Here's how the part is built. I have some questions about the finished solid (model axes, mm). Face numbers are marked on the shaded views. A direction names the side the tool comes from. Coordinates: 2 decimals unless noted, no trailing zeros. Loops run counter-clockwise (first coordinate to the right, second up) from the corner with the lowest first, then second, coordinate; pieces in that order, holes last. Notation, with made-up numbers: (87, -23) -> (109, -23) arc R19 ccw to (109, -8) -> close; hole circle Ø11 at (-16, 45.5). An arc over 180 degrees is marked (long way). Answer as a JSON object with one key per item and string values. Group by question number.
Q1. I want a section at D-D on y = -2.25. Write out the boundary of the cut face in (x, z).
Q2. I need wall thicknesses on line 1 (X direction, y = 0.5, z = 2.5); line 2 (X direction, y = -2.75, z = 1.45); line 3 (Y direction, x = 4.9, z = 1.7) (3 decimals). Which ranges of each line are inside material? Lowest first, please.
Q3. Thinking about a two-plate mould opening in X: for the marked faces 1, 2 and 3, which applies, released by +X, released by -X, zero draft, split by the parting line, or undercut?
Q4. I want a section at C-C on z = 1.2. Write out the boundary of the cut face in (x, y) (3 decimals), then the cut area to 3 significant figures.
Q5. I want a section at A-A on y = 0.95. Write out the boundary of the cut face in (x, z) (3 decimals).
Q6. I want a section at B-B on x = -4.9. Write out the boundary of the cut face in (y, z) (3 decimals), then the cut area to 4 significant figures.
Q7. I'm going to push flat-ended pins straight in: pin 1 (3 mm diameter, centred on x = 4.9, y = 0.95, fed in from +Z); pin 2 (1.6 mm diameter, centred on x = 0, z = 1, fed in from -Y). Where does each tip first touch, or does it pass through?
Q8. On a 3-axis mill with a long thin cutter (end or side, diameter ignored), from which of +Z, -Z, +X, -X, +Y, -Y can I reach the whole of each face in a straight line? I mean the marked faces 4 and 5. Say none if no direction works.
```python
from build123d import *

# Parameters (mm, degrees)
SKETCH1_W           = 20.2
SKETCH1_H           = 7.4
SKETCH1_R           = 1.725
BOSS_EXTRUDE1_DEPTH = 3
SKETCH2_W           = 2
SKETCH2_H           = 6
CUT_EXTRUDE1_DEPTH  = 3
FILLET1_R           = 1


with BuildPart() as part:
    # Sketch1 → Boss-Extrude1 (new body)
    with BuildSketch(Plane.XY):
        Rectangle(SKETCH1_W, SKETCH1_H)
        with Locations((-4.9, 0.95)):
            Circle(SKETCH1_R, mode=Mode.SUBTRACT)
        with Locations((4.9, 0.95)):
            Circle(SKETCH1_R, mode=Mode.SUBTRACT)
    extrude(amount=BOSS_EXTRUDE1_DEPTH)

    # Sketch2 → Cut-Extrude1 (cut)
    with BuildSketch(Plane.XY.offset(3)):
        with Locations((0, -0.7)):
            Rectangle(SKETCH2_W, SKETCH2_H)
    extrude(amount=-CUT_EXTRUDE1_DEPTH, mode=Mode.SUBTRACT)

    # Fillet1
    fillet1_edges = [part.edges().sort_by_distance(p)[0] for p in [
        (-10.1, 3.7, 1.5),
        (10.1, 3.7, 1.5),
    ]]
    fillet(fillet1_edges, radius=FILLET1_R)


solid = part.part
```
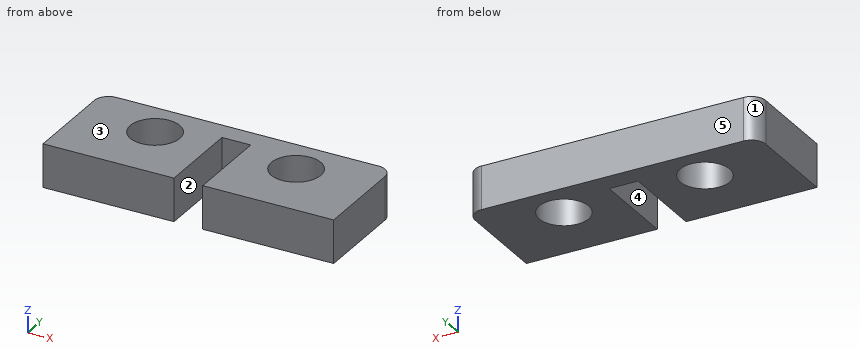
Result set:
{
 "1": {"outline": "(-10.1, 0) -> (-1, 0) -> (-1, 3) -> (-10.1, 3) -> close; (1, 0) -> (10.1, 0) -> (10.1, 3) -> (1, 3) -> close"},
 "2": {"line 1": "x = -10.1 to -6.57, -3.23 to -1, 1 to 3.23, 6.57 to 10.1", "line 2": "x = -10.1 to -1, 1 to 10.1", "line 3": "y = -3.7 to -0.775, 2.675 to 3.7"},
 "3": {"face 1": "released by -X", "face 2": "undercut", "face 3": "zero draft"},
 "4": {"outline": "(-10.1, -3.7) -> (-1, -3.7) -> (-1, 2.3) -> (1, 2.3) -> (1, -3.7) -> (10.1, -3.7) -> (10.1, 2.7) arc R1 ccw to (9.1, 3.7) -> (-9.1, 3.7) arc R1 ccw to (-10.1, 2.7) -> close; hole circle Ø3.45 at (-4.9, 0.95); hole circle Ø3.45 at (4.9, 0.95)", "area": "118 mm²"},
 "5": {"outline": "(-10.1, 0) -> (-6.625, 0) -> (-6.625, 3) -> (-10.1, 3) -> close; (-3.175, 0) -> (-1, 0) -> (-1, 3) -> (-3.175, 3) -> close; (1, 0) -> (3.175, 0) -> (3.175, 3) -> (1, 3) -> close; (6.625, 0) -> (10.1, 0) -> (10.1, 3) -> (6.625, 3) -> close"},
 "6": {"outline": "(-3.7, 0) -> (-0.775, 0) -> (-0.775, 3) -> (-3.7, 3) -> close; (2.675, 0) -> (3.7, 0) -> (3.7, 3) -> (2.675, 3) -> close", "area": "11.85 mm²"},
 "7": {"pin 1": "passes through", "pin 2": "stops at y = 2.3"},
 "8": {"face 4": "+Z, -Z, -Y", "face 5": "+Z, -Z, +X, -X, +Y"}
}
